The listing builds one solid part. Answer for the finished solid, in the listing's coordinates (mm). A direction names the side the tool comes from. Coordinates: 2 decimals unless noted, no trailing zeros. Order: outer loops, then holes, each group sorted by start corner. A loop starts at its lowest first (then second) coordinate and runs counter-clockwise, first axis right, second up. Notation, with made-up numbers: (-36, 2) -> (-18, 2) arc R24 cw to (-18, 22) -> close; hole circle Ø6 at (-31.5, 5.25). An arc over 180 degrees is marked (long way). Answer in a Markdown table with one row per item.
```python
from build123d import *

# Parameters (mm, degrees)
ESQUISSE1_W             = 10
ESQUISSE1_H             = 20
ESQUISSE1_R             = 2
BOSS_EXTRU_1_DEPTH      = 8
ESQUISSE2_R             = 2.65
ENL_V_MAT_EXTRU_1_DEPTH = 5
CONG_1_R                = 5


with BuildPart() as part:
    # Esquisse1 → Boss.-Extru.1 (new body)
    with BuildSketch(Plane(origin=(0, 0, 0), x_dir=(1, 0, 0), z_dir=(0, 1, 0))):
        with Locations((5, 10)):
            Rectangle(ESQUISSE1_W, ESQUISSE1_H)
        with Locations(Location((5, 16, 0), (0, 0, 270))):
            Circle(ESQUISSE1_R, mode=Mode.SUBTRACT)
        with Locations(Location((5, 4, 0), (0, 0, 90))):
            Circle(ESQUISSE1_R, mode=Mode.SUBTRACT)
    extrude(amount=BOSS_EXTRU_1_DEPTH)

    # Esquisse2 → Enlèv. mat.-Extru.1 (cut)
    with BuildSketch(Plane(origin=(0, 8, 0), x_dir=(1, 0, 0), z_dir=(0, 1, 0))):
        with Locations(Location((5, 10, 0), (0, 0, 270))):
            Circle(ESQUISSE2_R)
    extrude(amount=-ENL_V_MAT_EXTRU_1_DEPTH, mode=Mode.SUBTRACT)

    # Congé1
    cong_1_edges = [part.edges().sort_by_distance(p)[0] for p in [
        (0, 4, 0),
        (10, 4, 0),
        (0, 4, -20),
        (10, 4, -20),
    ]]
    fillet(cong_1_edges, radius=CONG_1_R - 0.0001)  # a hair under: the kernel refuses the full size


solid = part.part
```
(1) A cutting plane is placed at D-D, the plane x = 3.5. Determine the outline of the cut face in (y, z), then the cut area to 3 significant figures.
Check values:
| item | result |
|---|---|
| outline | (0, -19.77) -> (8, -19.77) -> (8, -17.32) -> (0, -17.32) -> close; (0, -14.68) -> (8, -14.68) -> (8, -12.18) -> (3, -12.18) -> (3, -7.82) -> (8, -7.82) -> (8, -5.32) -> (0, -5.32) -> close; (0, -2.68) -> (8, -2.68) -> (8, -0.23) -> (0, -0.23) -> close |
| area | 92.1 mm² |
(2) For a pull along X with two mould halves and no side action, classify faces 3 (the cylindrical face through (5, 4, -18)), 4 (the cylindrical face through (1, 4, -2)), 5 (the cylindrical face through (3.388, 5.535, -12.103)), 6 (the flat face through (10, 4, -10)) as released by +X, released by -X, zero draft, split by the parting line, or undercut.
Check values:
| item | result |
|---|---|
| face 3 | undercut |
| face 4 | released by -X |
| face 5 | undercut |
| face 6 | released by +X |
(3) A cutting plane is placed at B-B, the plane z = -16. Determine the outline of the cut face in (x, y), then the cut area to 3 significant figures.
Check values:
| item | result |
|---|---|
| outline | (0.1, 0) -> (3, 0) -> (3, 8) -> (0.1, 8) -> close; (7, 0) -> (9.9, 0) -> (9.9, 8) -> (7, 8) -> close |
| area | 46.4 mm² |
(4) A cutting plane is placed at A-A, the plane y = 5.5. Count the separate pieces of the cut face and the enclosed holes in it, then the cut area to 3 significant figures.
Check values:
| item | result |
|---|---|
| separate pieces | 1 |
| enclosed holes | 3 |
| area | 131 mm² |
(5) A cutting plane is placed at C-C, the plane z = -10. Determine the outline of the cut face in (x, y), then the cut area to 3 significant figures.
Check values:
| item | result |
|---|---|
| outline | (0, 0) -> (10, 0) -> (10, 8) -> (7.65, 8) -> (7.65, 3) -> (2.35, 3) -> (2.35, 8) -> (0, 8) -> close |
| area | 53.5 mm² |
(6) Which of the six approach directions +Z, -Z, +X, -X, +Y, -Y give full straight-line access (tool end or side, diameter ignored) to faces 1 (the flat face through (5, 3, -10)), 2 (the cylindrical face through (6.2, 3.9, -2.4))?
Check values:
| item | result |
|---|---|
| face 1 | +Y |
| face 2 | +Y, -Y |
(7) Flat-ended cylindrical pins translate along their axes: pin 1 (2.5 mm diameter, centred on x = 5, z = -10, fed in from +Y); pin 2 (5 mm diameter, centred on x = 5, z = -10, fed in from -Y); pin 3 (1.5 mm diameter, centred on y = 1.5, z = -3.5, fed in from -X); pin 4 (2 mm diameter, centred on x = 9, y = 6, fed in from -Z). Find the tip coordinate at first contact, or state that the pin passes through.
Check values:
| item | result |
|---|---|
| pin 1 | y = 3 |
| pin 2 | y = 0 |
| pin 3 | x = 0.06 |
| pin 4 | z = -19 |
(8) Find the intervals of material crossed by line 1 along Z through (x, y) = (3.25, 5.5); line 2 along X through (y, z) = (5.9, -10); line 3 along Z through (x, y) = (5.5, 7.25), in increasing order. Write a range as from..to.
Check values:
| item | result |
|---|---|
| line 1 | -19.68..-16.97, -15.03..-11.99, -8.01..-4.97, -3.03..-0.32 |
| line 2 | 0..2.35, 7.65..10 |
| line 3 | -19.97..-17.94, -14.06..-12.6, -7.4..-5.94, -2.06..-0.03 |
